from build123d import *

# Parameters (mm, degrees)
BOSS_EXTRU_1_DEPTH      = 10.5
ESQUISSE2_R             = 1.5
ENL_V_MAT_EXTRU_1_DEPTH = 11.5
CONG_1_R                = 3
ESQUISSE3_W             = 18
ESQUISSE3_H             = 10.5
BOSS_EXTRU_2_DEPTH      = 0.01
ESQUISSE4_R             = 1.5
BOSS_EXTRU_3_DEPTH      = 300


with BuildPart() as part:
    # Esquisse1 → Boss.-Extru.1 (new body)
    with BuildSketch(Plane.XY):
        Polygon((0, 0), (31, 0), (31, 20), (7, 20), (0, 13), align=None)
    extrude(amount=-BOSS_EXTRU_1_DEPTH)

    # Esquisse2 → Enlèv. mat.-Extru.1 (cut, through all)
    with BuildSketch(Plane.XY):
        with Locations((3, 3)):
            Circle(ESQUISSE2_R)
        with Locations((28, 3)):
            Circle(ESQUISSE2_R)
    extrude(amount=-ENL_V_MAT_EXTRU_1_DEPTH, mode=Mode.SUBTRACT)

    # Congé1
    cong_1_edges = [part.edges().sort_by_distance(p)[0] for p in [
        (31, 0, -5.25),
        (0, 0, -5.25),
    ]]
    fillet(cong_1_edges, radius=CONG_1_R)

    # Esquisse3 → Boss.-Extru.2 (add)
    with BuildSketch(Plane.XZ):
        with Locations((15.5, -5.25)):
            Rectangle(ESQUISSE3_W, ESQUISSE3_H)
    extrude(amount=BOSS_EXTRU_2_DEPTH)

    # Esquisse4 → Boss.-Extru.3 (add)
    with BuildSketch(Plane.XZ.offset(0.01)):
        with Locations((15.5, -5.25)):
            Circle(ESQUISSE4_R)
    extrude(amount=BOSS_EXTRU_3_DEPTH)


solid = part.part
The model under review builds one solid part; all positions refer to its coordinate system, in mm. Coordinates: 2 decimals unless noted, no trailing zeros. Write each loop counter-clockwise with the first axis right and the second up, starting at its lowest first coordinate (ties: lowest second). Pieces come first, ordered by that corner, then holes. Notation, with made-up numbers: (68.25, 46) - (103.25, 46) arc R17 cw to (103.25, 56) - close; hole circle Ø4 at (-4, -28). An arc over 180 degrees is marked (long way). Answer as CSV lines item,"result".
(1) For line 1 along Y through (x, z) = (28, -7); line 2 along Y through (x, z) = (29, -7.75); line 3 along X through (y, z) = (-51.5, -5.5), list the stretches that pass through material, from the lowest coordinate up. Write a range as [from, to].
Data:
line 1,"y = [0, 1.5], [4.5, 20]"
line 2,"y = [0.17, 1.88], [4.12, 20]"
line 3,"x = [14.02, 16.98]"
(2) Clearance check with flat-ended pins moving along their axes: pin 1 Ø1 at (x, z) = (26, -7.5) entering from -Y; pin 2 Ø1 at (x, y) = (15.5, -181) entering from -Z; pin 3 Ø6 at (y, z) = (-49.5, -7.5) entering from -X. State where each tip first meets the part, or that it passes through.
Data:
pin 1,"stops at y = 0"
pin 2,"stops at z = -6.75"
pin 3,"stops at x = 14"
(3) We need section A-A (z = -8.5). Count the separate pieces of the cut face and the enclosed holes in it, plus the area to 3 significant figures.
Data:
separate pieces,"1"
enclosed holes,"2"
area,"578 mm2"
(4) We need section B-B (y = -71). Give the boundary of the cut face in (x, z).
Data:
outline,"circle Ø3 at (15.5, -5.25)"
